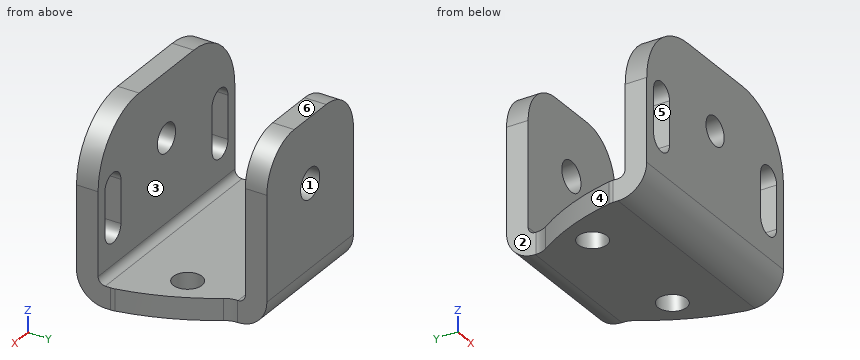
from build123d import *

# Parameters (mm, degrees)
BRIDA_BASE1_DEPTH                = 3
BRIDA_DE_ARISTA1_STRIP_W         = 14
BRIDA_DE_ARISTA1_STRIP_H         = 3
BRIDA_DE_ARISTA1_STRIP_CUT_DEPTH = 30
BRIDA_DE_ARISTA1_DEPTH           = 30
BRIDA_DE_ARISTA2_DEPTH           = 19
CORTAR_EXTRUIR1_REACH            = 45.489
CROQUIS12_R                      = 2
CORTAR_EXTRUIR2_REACH            = 43.979
CORTAR_EXTRUIR6_REACH            = 45.592
CROQUIS26_R                      = 2
TALADRO_ROSCADO_M51_D            = 4.2
TALADRO_ROSCADO_M51_DEPTH        = 3
REDONDEO2_R                      = 9
REDONDEO3_R                      = 6
REDONDEO4_R                      = 3


# Sheet-metal steps are written as plain solids
with BuildPart() as part:
    # Croquis1 → Brida base1 (new body)
    with BuildSketch(Plane.XY):
        with BuildLine():
            Line((0, 0), (30, 0))
            Line((30, 0), (30, 2))
            ThreePointArc((30, 2), (27.949996593, 8.796152405), (24.5, 15))
            Line((24.5, 15), (24.5, 16))
            Line((24.5, 16), (5.5, 16))
            Line((5.5, 16), (5.5, 15))
            ThreePointArc((5.5, 15), (2.050003407, 8.796152405), (0, 2))
            Line((0, 2), (0, 0))
        make_face()
    extrude(amount=-BRIDA_BASE1_DEPTH)

    # Brida de arista1 strip (across the edge) → Brida de arista1 strip cut (cut)
    with BuildSketch(Plane.YZ):
        with Locations((-6, -1.5)):
            Rectangle(BRIDA_DE_ARISTA1_STRIP_W, BRIDA_DE_ARISTA1_STRIP_H)
    extrude(amount=BRIDA_DE_ARISTA1_STRIP_CUT_DEPTH, mode=Mode.SUBTRACT)

    # Brida de arista1 section (across the edge) → Brida de arista1 (add)
    with BuildSketch(Plane.YZ):
        with BuildLine():
            Line((-3, 1), (-3, 21.5))
            Line((-3, 21.5), (0, 21.5))
            Line((0, 21.5), (0, 1))
            ThreePointArc((0, 1), (0.292893219, 0.292893219), (1, 0))
            Line((1, 0), (1, -3))
            ThreePointArc((1, -3), (-1.828427125, -1.828427125), (-3, 1))
        make_face()
    extrude(amount=BRIDA_DE_ARISTA1_DEPTH)

    # Brida de arista2 section (across the edge) → Brida de arista2 (add)
    with BuildSketch(Plane(origin=(24.5, 17, 0), x_dir=(0, -1, 0), z_dir=(-1, 0, 0))):
        with BuildLine():
            Line((-3, 1), (-3, 21.5))
            Line((-3, 21.5), (0, 21.5))
            Line((0, 21.5), (0, 1))
            ThreePointArc((0, 1), (0.292893219, 0.292893219), (1, 0))
            Line((1, 0), (1, -3))
            ThreePointArc((1, -3), (-1.828427125, -1.828427125), (-3, 1))
        make_face()
    extrude(amount=BRIDA_DE_ARISTA2_DEPTH)

    # Croquis12 → Cortar-Extruir1 (cut, up to next)
    with BuildSketch(Plane(origin=(0, -3, 0), x_dir=(1, 0, 0), z_dir=(0, 1, 0)), mode=Mode.PRIVATE) as cortar_extruir1_sk1:
        with Locations(Location((15, -12.5, 0), (0, 0, 270))):
            Circle(CROQUIS12_R)
    cortar_extruir1_tool1 = extrude(cortar_extruir1_sk1.sketch, amount=CORTAR_EXTRUIR1_REACH, mode=Mode.PRIVATE) & part.part
    add(cortar_extruir1_tool1.solids().sort_by_distance((15, -3, 12.5))[0], mode=Mode.SUBTRACT)

    # Croquis13 → Cortar-Extruir2 (cut, up to next)
    with BuildSketch(Plane(origin=(0, 0, 0), x_dir=(1, 0, 0), z_dir=(0, 1, 0)), mode=Mode.PRIVATE) as cortar_extruir2_sk1:
        with BuildLine():
            Line((5, -5.75), (5, -11.75))
            ThreePointArc((5, -11.75), (3.25, -13.5), (1.5, -11.75))
            Line((1.5, -11.75), (1.5, -5.75))
            ThreePointArc((1.5, -5.75), (3.25, -4), (5, -5.75))
        make_face()
    cortar_extruir2_tool1 = extrude(cortar_extruir2_sk1.sketch, amount=-CORTAR_EXTRUIR2_REACH, mode=Mode.PRIVATE) & part.part
    # Croquis13 → Cortar-Extruir2 (cut, up to next)
    with BuildSketch(Plane(origin=(0, 0, 0), x_dir=(1, 0, 0), z_dir=(0, 1, 0)), mode=Mode.PRIVATE) as cortar_extruir2_sk2:
        with BuildLine():
            Line((25, -5.75), (25, -11.75))
            ThreePointArc((25, -11.75), (26.75, -13.5), (28.5, -11.75))
            Line((28.5, -11.75), (28.5, -5.75))
            ThreePointArc((28.5, -5.75), (26.75, -4), (25, -5.75))
        make_face()
    cortar_extruir2_tool2 = extrude(cortar_extruir2_sk2.sketch, amount=-CORTAR_EXTRUIR2_REACH, mode=Mode.PRIVATE) & part.part
    add(cortar_extruir2_tool1.solids().sort_by_distance((3.25, 0, 8.75))[0], mode=Mode.SUBTRACT)
    add(cortar_extruir2_tool2.solids().sort_by_distance((26.75, 0, 8.75))[0], mode=Mode.SUBTRACT)

    # Croquis26 → Cortar-Extruir6 (cut, up to next)
    with BuildSketch(Plane(origin=(0, 0, -3), x_dir=(-1, 0, 0), z_dir=(0, 0, -1)), mode=Mode.PRIVATE) as cortar_extruir6_sk1:
        with Locations((-6.25, 8.5)):
            Circle(CROQUIS26_R)
    cortar_extruir6_tool1 = extrude(cortar_extruir6_sk1.sketch, amount=-CORTAR_EXTRUIR6_REACH, mode=Mode.PRIVATE) & part.part
    # Croquis26 → Cortar-Extruir6 (cut, up to next)
    with BuildSketch(Plane(origin=(0, 0, -3), x_dir=(-1, 0, 0), z_dir=(0, 0, -1)), mode=Mode.PRIVATE) as cortar_extruir6_sk2:
        with Locations((-23.75, 8.5)):
            Circle(CROQUIS26_R)
    cortar_extruir6_tool2 = extrude(cortar_extruir6_sk2.sketch, amount=-CORTAR_EXTRUIR6_REACH, mode=Mode.PRIVATE) & part.part
    add(cortar_extruir6_tool1.solids().sort_by_distance((6.25, 8.5, -3))[0], mode=Mode.SUBTRACT)
    add(cortar_extruir6_tool2.solids().sort_by_distance((23.75, 8.5, -3))[0], mode=Mode.SUBTRACT)

    # Taladro roscado M51
    with Locations(Plane(origin=(15, 20, 12.5), x_dir=(0, 0, 1), z_dir=(0, 1, 0))):
        with Locations((0, 0)):
            Hole(TALADRO_ROSCADO_M51_D / 2, depth=TALADRO_ROSCADO_M51_DEPTH)

    # Redondeo2
    redondeo2_edges = [part.edges().sort_by_distance(p)[0] for p in [
        (0, -1.5, 21.5),
        (30, -1.5, 21.5),
    ]]
    fillet(redondeo2_edges, radius=REDONDEO2_R)

    # Redondeo3
    redondeo3_edges = [part.edges().sort_by_distance(p)[0] for p in [
        (24.5, 18.5, 21.5),
        (5.5, 18.5, 21.5),
    ]]
    fillet(redondeo3_edges, radius=REDONDEO3_R)

    # Redondeo4
    redondeo4_edges = [part.edges().sort_by_distance(p)[0] for p in [
        (0, 2, -1.5),
        (5.5, 15, -1.5),
        (24.5, 15, -1.5),
        (30, 2, -1.5),
    ]]
    fillet(redondeo4_edges, radius=REDONDEO4_R)


solid = part.part
Input: part model. Units: mm. Frame: model coordinates. Face numbers are marked on the shaded views. A direction names the side the tool comes from. Coordinates: 2 decimals unless noted, no trailing zeros. Loops run counter-clockwise (first coordinate to the right, second up) from the corner with the lowest first, then second, coordinate; pieces in that order, holes last.
Q1. Material intervals for line 1 (X direction, y = -2, z = 9.25); line 2 (Y direction, x = 14.75, z = 14.75); line 3 (X direction, y = 17.95, z = 12.5), sorted ascending.
Q2. Cut plane C-C (y = 8.5). Output: boundary loops of the cut face in (x, z), then the cut area to 3 significant figures.
Q3. Cut plane D-D (x = 26.75). Output: boundary loops of the cut face in (y, z), then the cut area to 3 significant figures.
Q4. Draft query along X for the marked faces 4, 5 and 6. Return one class per face: +X half, -X half, draft (parallel to the pull), parting line (faces both ways), or undercut.
Q5. Cut plane B-B (z = 16.5). Output: boundary loops of the cut face in (x, y), then the cut area to 3 significant figures.
Q6. Cut plane A-A (x = 15). Output: boundary loops of the cut face in (y, z).
Q7. Set-up query: the marked faces 1, 2 and 3. Return all of +Z, -Z, +X, -X, +Y, -Y with unobstructed straight access to the full face (end or side cutting, diameter ignored); none if empty.
Q8. Contact query for flat-ended pins moving along their axis: pin 1 (4 mm diameter, centred on y = 17, z = 11, fed in from -X); pin 2 (6.5 mm diameter, centred on x = 6.25, y = 8.5, fed in from +Z); pin 3 (4.5 mm diameter, centred on y = 17, z = 2, fed in from +X). Output: stop coordinate, or through.
Working result:
1. line 1: x = 0 to 1.5, 5 to 25, 28.5 to 30
1. line 2: y = -3 to 0, 17 to 20
1. line 3: x = 5.5 to 12.9, 17.1 to 24.5
2. outline: (1.93, -3) - (4.25, -3) - (4.25, 0) - (1.93, 0) - close; (8.25, -3) - (21.75, -3) - (21.75, 0) - (8.25, 0) - close; (25.75, -3) - (28.07, -3) - (28.07, 0) - (25.75, 0) - close
2. area: 54.4 mm2
3. outline: (-3, 1) arc R4 ccw to (1, -3) - (11.33, -3) - (11.33, 0) - (1, 0) arc R1 cw to (0, 1) - (0, 4) - (-3, 4) - close; (-3, 13.5) - (0, 13.5) - (0, 19.42) - (-3, 19.42) - close
3. area: 69.5 mm2
4. face 4: -X half
4. face 5: undercut
4. face 6: draft
5. outline: (0.94, -3) - (29.06, -3) - (29.06, 0) - (0.94, 0) - close; (5.58, 17) - (24.42, 17) - (24.42, 20) - (5.58, 20) - close
5. area: 141 mm2
6. outline: (-3, 1) arc R4 ccw to (1, -3) - (16, -3) arc R4 ccw to (20, 1) - (20, 10.4) - (17, 10.4) - (17, 1) arc R1 cw to (16, 0) - (1, 0) arc R1 cw to (0, 1) - (0, 10.5) - (-3, 10.5) - close; (-3, 14.5) - (0, 14.5) - (0, 21.5) - (-3, 21.5) - close; (17, 14.6) - (20, 14.6) - (20, 21.5) - (17, 21.5) - close
7. face 1: +Y
7. face 2: +Z, -Z, -X, +Y
7. face 3: +Z, +X, -X
8. pin 1: stops at x = 5.5
8. pin 2: stops at z = 0
8. pin 3: stops at x = 24.5
